Check sheet for the modelled part. Datum: model origin and axes. Units: mm. Face numbers are marked on the shaded views. A direction names the side the tool comes from. Coordinates: 2 decimals unless noted, no trailing zeros. Write each loop counter-clockwise with the first axis right and the second up, starting at its lowest first coordinate (ties: lowest second). Pieces come first, ordered by that corner, then holes. Notation, with made-up numbers: (9.5, 72.5) - (49.5, 72.5) arc R30 ccw to (49.5, 98.5) - close; hole circle Ø8 at (66.25, 48). An arc over 180 degrees is marked (long way). Use one line per item in the form item = value. Start each with the question number.
1. Cross-section at A-A on x = 0. Record the boundary of the cut face in (y, z).
2. Go/stop test with flat-tipped pins: pin 1 Ø10 at (y, z) = (12, 3) entering from -X; pin 2 Ø1.5 at (x, z) = (-1.5, 13.5) entering from -Y; pin 3 Ø1.5 at (x, z) = (14.5, 4) entering from +Y. Record where each tip stops, or that it passes through.
3. Cross-section at D-D on x = -7. Record the boundary of the cut face in (y, z).
4. Draft check along X on the marked faces 4, 5 and 6. Enter one of: +X half, -X half, draft (parallel to the pull), parting line (faces both ways), or undercut.
5. Tool access check on the marked faces 1, 2 and 3. Record the directions out of +Z, -Z, +X, -X, +Y, -Y that give a thin tool (end or side, any length) a straight path to the whole face; none if there is none.
6. Scan lines: line 1 along Z through (x, y) = (-18, 6.5); line 2 along Y through (x, z) = (0, 8.5); line 3 along Z through (x, y) = (-14, 4). Record each from-to range of solid material in increasing order.
7. Cross-section at C-C on z = 9.75. Record the boundary of the cut face in (x, y), then the cut area to 3 significant figures.
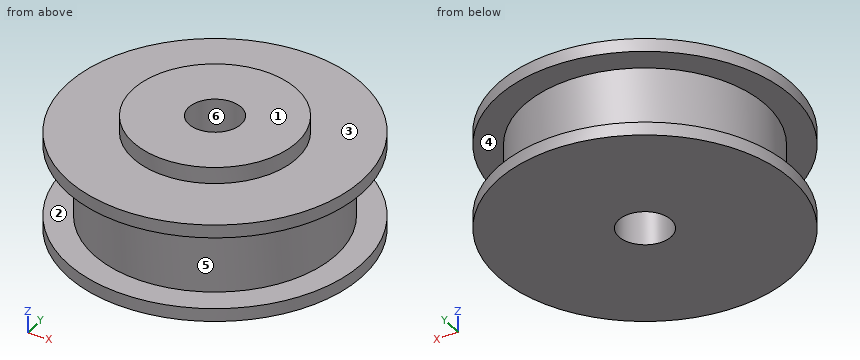
```python
from build123d import *

# Parameters (mm, degrees)
SKETCH_1_R          = 22.5
EXTRUDE_1_DEPTH     = 15
SKETCH_2_R          = 12.5
EXTRUDE_2_DEPTH     = 2.5
SKETCH_3_R          = 4
CUT_EXTRUDE_1_DEPTH = 45
SKETCH_5_W          = 4
SKETCH_5_H          = 11


with BuildPart() as part:
    # 草图1 → 凸台-拉伸1 (new body)
    with BuildSketch(Plane.XY):
        Circle(SKETCH_1_R)
    extrude(amount=EXTRUDE_1_DEPTH)

    # 草图2 → 凸台-拉伸2 (add)
    with BuildSketch(Plane.XY.offset(15)):
        Circle(SKETCH_2_R)
    extrude(amount=EXTRUDE_2_DEPTH)

    # 草图3 → 切除-拉伸1 (cut)
    with BuildSketch(Plane.XY.offset(17.5)):
        Circle(SKETCH_3_R)
    extrude(amount=-CUT_EXTRUDE_1_DEPTH, mode=Mode.SUBTRACT)

    # 草图5 → 切除-旋转1 (revolve, cut)
    with BuildSketch(Plane(origin=(0, 0, 0), x_dir=(1, 0, 0), z_dir=(0, 1, 0)), mode=Mode.PRIVATE) as cut_revolve_1_sk:
        with Locations((20.5, -7.5)):
            Rectangle(SKETCH_5_W, SKETCH_5_H)
    revolve(cut_revolve_1_sk.sketch.rotate(Axis((0, 0, 0), (0, 0, 1)), 180), axis=Axis((0, 0, 0), (0, 0, 1)), mode=Mode.SUBTRACT)


solid = part.part
```
Final values:
q1.outline = (-22.5, 0) - (-4, 0) - (-4, 17.5) - (-12.5, 17.5) - (-12.5, 15) - (-22.5, 15) - (-22.5, 13) - (-18.5, 13) - (-18.5, 2) - (-22.5, 2) - close; (4, 0) - (22.5, 0) - (22.5, 2) - (18.5, 2) - (18.5, 13) - (22.5, 13) - (22.5, 15) - (12.5, 15) - (12.5, 17.5) - (4, 17.5) - close
q2.pin_1 = -21.35
q2.pin_2 = -22.49
q2.pin_3 = 12.38
q3.outline = (-21.38, 0) - (21.38, 0) - (21.38, 2) - (17.12, 2) - (17.12, 13) - (21.38, 13) - (21.38, 15) - (10.36, 15) - (10.36, 17.5) - (-10.36, 17.5) - (-10.36, 15) - (-21.38, 15) - (-21.38, 13) - (-17.12, 13) - (-17.12, 2) - (-21.38, 2) - close
q4.face_4 = draft
q4.face_5 = parting line
q4.face_6 = undercut
q5.face_1 = +Z, +X, -X, +Y, -Y
q5.face_2 = none
q5.face_3 = +Z
q6.line_1 = 0 to 2, 13 to 15
q6.line_2 = -18.5 to -4, 4 to 18.5
q6.line_3 = 0 to 15
q7.outline = circle Ø37 at (0, 0); hole circle Ø8 at (0, 0)
q7.area = 1,020 mm²
